Design review of the part built by this model. Coordinates are the model's own, in mm. Face numbers are marked on the shaded views. A direction names the side the tool comes from. Give positions to 0.01 mm unless a question says otherwise; leave off trailing zeros. Loops run counter-clockwise (first coordinate to the right, second up) from the corner with the lowest first, then second, coordinate; pieces in that order, holes last. Notation, with made-up numbers: (23, 17) -> (46, 17) arc R24 cw to (46, 30) -> close; hole circle Ø6 at (85, 70). An arc over 180 degrees is marked (long way). Answer as CSV lines item,"result".
Autodesk Inventor part; units mm, degrees
ref_plane "Work Plane1" through (0, -10.5, 0) normal (0, 1, 0) x (-1, 0, 0)
ref_plane "YZ Plane" through (0, 0, 0) normal (1, 0, 0) x (0, 1, 0)
ref_plane "XY Plane" through (0, 0, 0) normal (0, 0, 1) x (1, 0, 0)
sketch "Sketch1" plane through (0, 0, 0) normal (0, 0, 1) x (1, 0, 0)
  circle A0 centre (0, 0) radius 1.825
  circle A1 centre (0, 0) radius 4.825
  line L0 (-6, -4) -> (6, -4)
  line L1 (6, -10.5) -> (-6, -10.5)
  line L2 (-6, -10.5) -> (-6, -4)
  arc A2 (-2.3662, -0.949) -> (-6, -4) centre (-3.6609, -3.0965) ccw
  arc A3 (6, -4) -> (2.3662, -0.949) centre (3.6609, -3.0965) ccw
  arc A4 (-2.3662, -0.949) -> (2.3662, -0.949) centre (0, 0.4878) ccw
  line L3 (-15.4666, 0) -> (16.043, 0) construction
  line L4 (0, 8.2762) -> (0, -10.4238) construction
  line L5 (6, -10.5) -> (6, -4)
  dimension "d0" = 3.65
  dimension "d1" = 3
  dimension "d3" = 12
  dimension "d5" = 4
  dimension "d6" = 6.5
  dimension "d7" = 6
extrude "Extrusion1" add sketch "Sketch1" along normal blind 9
ref_plane "Work Plane1" through (0, -10.5, 0) normal (0, 1, 0) x (-1, 0, 0)
extrude "Extrusion4" add sketch "Sketch1" along normal blind 14 contours A1 A3 A4 A2 | A2 A4 A3 A1 L0 | L0 A1
sketch "Sketch2" plane through (0, -10.5, 0) normal (0, 1, 0) x (-1, 0, 0)
  line L0 (6, 0) -> (-6, 0)
  line L1 (-6, 0) -> (-6, 9)
  line L2 (6, 9) -> (-6, 9)
  line L3 (6, 0) -> (6, 9)
  circle A0 centre (0, 4) radius 2.125
  point P0 (0, 0)
  dimension "d11" = 4.25
  dimension "d12" = 4
extrude "Extrusion2" cut sketch "Sketch2" along normal blind 8 contours A0
sketch "Sketch3" plane through (0, 0, 9) normal (0, 0, 1) x (1, 0, 0)
  line L0 (-6, -10.5) -> (6, -10.5)
  circle A0 centre (0, 0) radius 1.825
  line L1 (-4.45, -4.5) -> (4.45, -4.5)
  line L2 (4.45, -4.5) -> (4.45, -8.1)
  line L3 (4.45, -8.1) -> (-4.45, -8.1)
  line L4 (-4.45, -8.1) -> (-4.45, -4.5)
  point P0 (0, -8.1)
  point P1 (0, -10.5)
  dimension "d15" = 8.9
  dimension "d16" = 3.6
  dimension "d17" = 4.5
extrude "Extrusion3" cut sketch "Sketch3" along normal mid plane 30 contours L1 L2 L3 L4
equation "\"d4\" = 0.4"
properties part number "MotorAttachment2"
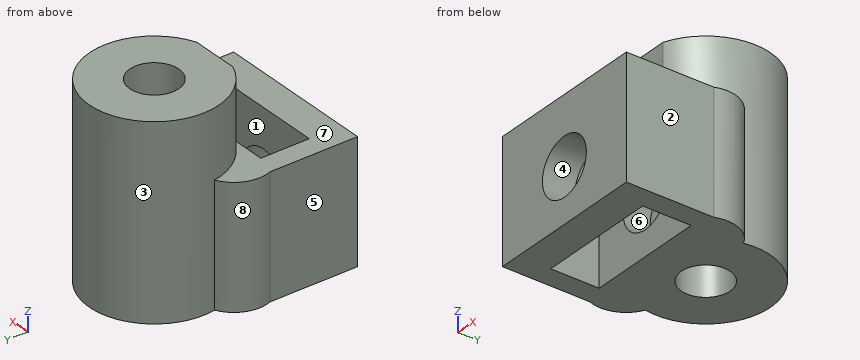
Q1. For the marked faces 1, 2, 3, 4 and 5, list the 3-axis set-ups (+Z, -Z, +X, -X, +Y, -Y) from which the entire face can be reached by the end or side of a thin tool; tool diameter is ignored.
Filled sheet:
face 1,"+Z, -Z"
face 2,"+Z, -Z, +X, -Y"
face 3,"+Z"
face 4,"-Y"
face 5,"+Z, -Z, -X, -Y"
Q2. To check wall thickness, follow probe 1 along Z at (x, y) = (0, -9.15) (3 decimals); probe 2 along Z at (x, y) = (0, -3.6) (3 decimals); probe 3 along Y at (x, z) = (0, 9.5) (3 decimals). State the ranges of each line that lie inside material, in increasing order. Write a range as from..to.
Filled sheet:
probe 1,"z = 0..1.875, 6.125..9"
probe 2,"z = 0..1.875, 6.125..14"
probe 3,"y = -4.5..-1.825, 1.825..4.825"
Q3. We need section B-B, the plane y = -6. State the section outline as (x, z) points.
Filled sheet:
outline,"(-6, 0) -> (-4.45, 0) -> (-4.45, 9) -> (-6, 9) -> close; (4.45, 0) -> (6, 0) -> (6, 9) -> (4.45, 9) -> close"
Q4. We need section A-A, the plane x = 0. State the section outline as (y, z) points (3 decimals).
Filled sheet:
outline,"(-10.5, 0) -> (-8.1, 0) -> (-8.1, 1.875) -> (-10.5, 1.875) -> close; (-10.5, 6.125) -> (-8.1, 6.125) -> (-8.1, 9) -> (-10.5, 9) -> close; (-4.5, 0) -> (-1.825, 0) -> (-1.825, 14) -> (-4.5, 14) -> (-4.5, 6.125) -> (-2.5, 6.125) -> (-2.5, 1.875) -> (-4.5, 1.875) -> close; (1.825, 0) -> (4.825, 0) -> (4.825, 14) -> (1.825, 14) -> close"
Q5. We need section D-D, the plane z = 4. State the section outline as (x, y) points (3 decimals), and give its area (3 significant figures).
Filled sheet:
outline,"(-6, -10.5) -> (-2.125, -10.5) -> (-2.125, -8.1) -> (-4.45, -8.1) -> (-4.45, -4.5) -> (-2.125, -4.5) -> (-2.125, -2.5) -> (2.125, -2.5) -> (2.125, -4.5) -> (4.45, -4.5) -> (4.45, -8.1) -> (2.125, -8.1) -> (2.125, -10.5) -> (6, -10.5) -> (6, -4) arc R2.508 ccw to (4.752, -0.839) arc R4.825 ccw (long way) to (-4.752, -0.839) arc R2.508 ccw to (-6, -4) -> close; hole circle Ø3.65 at (0, 0)"
area,"98.5 mm^2"
Q6. Clearance check with flat-ended pins moving along their axes: pin 1 Ø3 at (y, z) = (-4, 11) entering from +X; pin 2 Ø2 at (y, z) = (-9, 5) entering from -X; pin 3 Ø1.5 at (y, z) = (3, 4) entering from +X; pin 4 Ø1 at (x, y) = (-3, -6.5) entering from +Z. State where each tip first meets the part, or that it passes through.
Filled sheet:
pin 1,"stops at x = 4.13"
pin 2,"stops at x = -6"
pin 3,"stops at x = 4.27"
pin 4,"passes through"
Q7. The part is to be moulded in two halves that separate along Z. For the marked faces 6, 7 and 8, say which applies: pulls with the +Z half, pulls with the -Z half, needs draft (parallel to the pull), parting line crosses it, or undercut.
Filled sheet:
face 6,"undercut"
face 7,"pulls with the +Z half"
face 8,"needs draft"
Q8. We need section C-C, the plane z = 6.5. State the section outline as (x, y) points (3 decimals), and give its area (3 significant figures).
Filled sheet:
outline,"(-6, -10.5) -> (6, -10.5) -> (6, -4) arc R2.508 ccw to (4.752, -0.839) arc R4.825 ccw (long way) to (-4.752, -0.839) arc R2.508 ccw to (-6, -4) -> close; hole (-4.45, -8.1) -> (4.45, -8.1) -> (4.45, -4.5) -> (-4.45, -4.5) -> close; hole circle Ø3.65 at (0, 0)"
area,"117 mm^2"
